from build123d import *

# Parameters (mm, degrees)
F1_DEPTH = 241.935
F2_R     = 38.1
F3_DEPTH = 38.1000004709
F4_R     = 63.5
F5_DEPTH = 38.1000004709
F6_R     = 190.5


with BuildPart() as f1:
    # F0 (on Right) → F1 (new body, symmetric)
    with BuildSketch(Plane.YZ):
        with BuildLine():
            Line((0, 0), (1270, 0))
            Line((1270, 0), (1270, 38.1000004709))
            Line((1270, 38.1000004709), (0, 38.1000004709))
            ThreePointArc((0, 38.1000004709), (-68.0529659297, 83.5715385522), (-52.0854851692, 163.8454851692))
            Line((-52.0854851692, 163.8454851692), (296.2988816537, 512.2298519922))
            Line((296.2988816537, 512.2298519922), (269.3581129575, 539.1706206883))
            Line((269.3581129575, 539.1706206883), (-79.0262538654, 190.7862538654))
            ThreePointArc((-79.0262538654, 190.7862538654), (-103.2527765535, 68.9912995989), (0, 0))
        make_face()
    extrude(amount=F1_DEPTH, both=True)

    # F2 (on face) → F3 (cut, through all)
    with BuildSketch(Plane(origin=(0, -134.9062538654, 134.9062538654), x_dir=(1, 0, 0), z_dir=(0, -0.7071067812, 0.7071067812))):
        with Locations((-127.635, 419.2442297935)):
            Circle(F2_R)
        with Locations((127.635, 419.2442297935)):
            Circle(F2_R)
    extrude(amount=-F3_DEPTH, mode=Mode.SUBTRACT)

    # F4 (on face) → F5 (cut, through all)
    with BuildSketch(Plane.XY.offset(38.1000004709)):
        with Locations((0, 457.2)):
            Circle(F4_R)
        with BuildLine():
            Line((-50.5338093541, 1100.8937581723), (-50.5338093541, 829.5062418277))
            ThreePointArc((-50.5338093541, 829.5062418277), (0, 774.7), (50.5338093541, 829.5062418277))
            Line((50.5338093541, 829.5062418277), (50.5338093541, 1100.8937581723))
            ThreePointArc((50.5338093541, 1100.8937581723), (0, 1155.7), (-50.5338093541, 1100.8937581723))
        make_face()
    extrude(amount=-F5_DEPTH, mode=Mode.SUBTRACT)

    # F6
    f6_edges = [f1.edges().sort_by_distance(p)[0] for p in [
        (-241.935, 282.828497, 525.700236),
        (241.935, 282.828497, 525.700236),
    ]]
    fillet(f6_edges, radius=F6_R)


solid = f1.part
Work out the finished part from the listing and answer in its coordinate system (mm). A direction names the side the tool comes from. Give positions to 0.01 mm unless a question says otherwise; leave off trailing zeros. Order: outer loops, then holes, each group sorted by start corner. A loop starts at its lowest first (then second) coordinate and runs counter-clockwise, first axis right, second up. Notation, with made-up numbers: M 46,67.5 L 66,67.5 A24 ccw 66,83.5 Z; hole C -13.5,37.25 d4. An arc over 180 degrees is marked long. Return JSON: item names as keys, results as strings.
Q1. The mould has two halves that part along Y. Classify faces 1 (the face through (50.534, 963, 19)), 2 (the face through (-187.612, 242.133, 485.382)), 3 (the face through (-241.935, 422, 23)): pulls with the +Y half, pulls with the -Y half, needs draft (parallel to the pull), parting line crosses it, or undercut.
Answer below:
{"face 1": "undercut", "face 2": "pulls with the +Y half", "face 3": "needs draft"}
Q2. Find section C-C, the plane x = -122.5. Write down the section's boundary in (y, z).
Answer below:
{"outline": "M -79.03,190.79 A111.76 ccw 0,0 L 1270,0 L 1270,38.1 L 0,38.1 A73.66 cw -52.09,163.85 L 161.79,377.72 L 134.85,404.66 Z; M 188.24,458.05 L 215.18,431.11 L 286.58,502.51 L 259.63,529.45 Z"}
Q3. Which of the six approach directions +Z, -Z, +X, -X, +Y, -Y give full straight-line access (tool end or side, diameter ignored) to faces 4 (the face through (0.72, 283.02, 525.51)), 5 (the face through (-50.534, 967, 19)), 6 (the face through (3.39, 119.67, 335.6))?
Answer below:
{"face 4": "+Z, +X, -X, +Y", "face 5": "+Z, -Z", "face 6": "+X, -X, +Y"}
Q4. Find section A-A, the plane y = 457.2. Write down the section's boundary in (x, z) (3 decimals).
Answer below:
{"outline": "M -241.935,0 L -63.5,0 L -63.5,38.1 L -241.935,38.1 Z; M 63.5,0 L 241.935,0 L 241.935,38.1 L 63.5,38.1 Z"}
Q5. Find section B-B, the plane x = 0. Write down the section's boundary in (y, z).
Answer below:
{"outline": "M -79.03,190.79 A111.76 ccw 0,0 L 393.7,0 L 393.7,38.1 L 0,38.1 A73.66 cw -52.09,163.85 L 296.3,512.23 L 269.36,539.17 Z; M 520.7,0 L 774.7,0 L 774.7,38.1 L 520.7,38.1 Z; M 1155.7,0 L 1270,0 L 1270,38.1 L 1155.7,38.1 Z"}
Q6. Find the intervals of material crossed by line 1 along Y through (x, z) = (0, 13); line 2 along Y through (x, z) = (0, 13.5); line 3 along Z through (x, y) = (54, 905), in increasing order. Write a range as [from, to].
Answer below:
{"line 1": "y = [-52.31, 393.7], [520.7, 774.7], [1155.7, 1270]", "line 2": "y = [-53.25, 393.7], [520.7, 774.7], [1155.7, 1270]", "line 3": "z = [0, 38.1]"}
Q7. Each of these flat-tipped pins is pushed along its axis until it touches: pin 1 (1.5 mm diameter, centred on x = 183.5, z = 95.5, fed in from +Y); pin 2 (8 mm diameter, centred on x = 188.5, z = 300.5, fed in from -Y); pin 3 (8 mm diameter, centred on x = -13, y = 88, fed in from +Z). Where does it stop, or does it pass through?
Answer below:
{"pin 1": "stops at y = -71.67", "pin 2": "stops at y = 26.69", "pin 3": "stops at z = 361.81"}
Q8. Find section D-D, the plane y = 637. Write down the section's boundary in (x, z) (3 decimals).
Answer below:
{"outline": "M -241.935,0 L 241.935,0 L 241.935,38.1 L -241.935,38.1 Z"}
